```python
from build123d import *

# Parameters (mm, degrees)
F0_W     = 300
F0_H     = 200
F0_R     = 25
F1_DEPTH = 40


with BuildPart() as f1:
    # F0 (on Front) → F1 (new body, symmetric)
    with BuildSketch(Plane.XZ):
        with Locations((-150, 0)):
            Rectangle(F0_W, F0_H)
        with Locations((-250, 0)):
            Circle(F0_R, mode=Mode.SUBTRACT)
    extrude(amount=F1_DEPTH, both=True)

    # F4: F1 across face


with BuildPart() as f2_1:
    # F2: instance of F1
    add(f1.part.mirror(Plane.YZ))


with BuildPart() as f1_1:
    add(f1.part)
    add(f1.part.mirror(Plane.YZ))


solid = f1_1.part
```
The model under review builds one solid part; all positions refer to its coordinate system, in mm. Round coordinates to 2 decimals unless told otherwise and drop trailing zeros. Write each loop counter-clockwise with the first axis right and the second up, starting at its lowest first coordinate (ties: lowest second). Pieces come first, ordered by that corner, then holes. Notation, with made-up numbers: (85.25, -35.5) - (124.25, -35.5) arc R5 cw to (124.25, -29.5) - close; hole circle Ø7 at (-14, 81). An arc over 180 degrees is marked (long way). Use one line per item in the form item = value.
Q1. Consider section A-A (x = -250). State the section outline as (y, z) points.
Answer key:
outline = (-40, -100) - (40, -100) - (40, -25) - (-40, -25) - close; (-40, 25) - (40, 25) - (40, 100) - (-40, 100) - close
Q2. Consider section D-D (x = 252.5). State the section outline as (y, z) points.
Answer key:
outline = (-40, -100) - (40, -100) - (40, -24.87) - (-40, -24.87) - close; (-40, 24.87) - (40, 24.87) - (40, 100) - (-40, 100) - close
Q3. Consider section B-B (z = 0). State the section outline as (x, y) points, and give its area (3 significant figures).
Answer key:
outline = (-300, -40) - (-275, -40) - (-275, 40) - (-300, 40) - close; (-225, -40) - (225, -40) - (225, 40) - (-225, 40) - close; (275, -40) - (300, -40) - (300, 40) - (275, 40) - close
area = 40,000 mm2
Q4. Consider section C-C (y = 13). State the section outline as (x, z) points.
Answer key:
outline = (-300, -100) - (300, -100) - (300, 100) - (-300, 100) - close; hole circle Ø50 at (-250, 0); hole circle Ø50 at (250, 0)
Q5. For line 1 (Z direction, x = -250, y = 13), list the stretches that pass through material, from the lowest coordinate up. Write a range as [from, to].
Answer key:
line_1 = [-100, -25], [25, 100]
Q6. Draft analysis for pull direction Z (two halves, no side actions). For faces 1 (the flat face through (4, -1, 100)), 2 (the cylindrical face through (-226.154, 0.56, 7.509)), 3 (the flat face through (-300, -1, -1)), state which applies: +Z half, -Z half, draft (parallel to the pull), parting line (faces both ways), or undercut.
Answer key:
face_1 = +Z half
face_2 = undercut
face_3 = draft
